from build123d import *

# Parameters (mm, degrees)
F1_DEPTH = 1.5
F3_DEPTH = 25
F4_R     = 0.5
F5_DEPTH = 2.5


# Not quite as in the source:
# - a feature names something its author has since deleted; it is built from what else it names


with BuildPart() as f1:
    # F0 (on Top) → F1 (new body)
    with BuildSketch(Plane.XY):
        Polygon((-37.5444034434, -27.2088618949), (12.4555965566, -35.5019792914), (22.4555965566, -35.5019792914), (22.4555965566, -18.9157444984), (12.4555965566, -18.9157444984), align=None)
    extrude(amount=F1_DEPTH)

    # F2 (on face) → F3 (join)
    with BuildSketch(Plane.XY.offset(1.5)):
        Polygon((-37.5444034434, -27.2088618949), (-1.9112733802, -33.1190565113), (-1.9112733802, -31.1190565113), (-25.486211666, -27.2088618949), (-1.9112733802, -23.2986672785), (-1.9112733802, -21.2986672785), align=None)
    extrude(amount=F3_DEPTH)

    # F4 (on face) → F5 (join)
    with BuildSketch(Plane.XY.offset(1.5)):
        with Locations((17.4555965566, -27.2088618949)):
            Circle(F4_R)
    extrude(amount=F5_DEPTH)


solid = f1.part
Model file for the job. Use its own axes, mm. A direction names the side the tool comes from. Give positions to 0.01 mm unless a question says otherwise; leave off trailing zeros. Write each loop counter-clockwise with the first axis right and the second up, starting at its lowest first coordinate (ties: lowest second). Pieces come first, ordered by that corner, then holes. Notation, with made-up numbers: (-13, 12) -> (11, 12) arc R17 ccw to (11, 27) -> close; hole circle Ø4 at (39, 70). An arc over 180 degrees is marked (long way). Write item = value, one per line.
(1) Slice it at A-A, the plane z = 10.25. Give the cut face in (x, y), then the cut area to 3 significant figures.
Determined:
outline = (-37.54, -27.21) -> (-1.91, -33.12) -> (-1.91, -31.12) -> (-25.49, -27.21) -> (-1.91, -23.3) -> (-1.91, -21.3) -> close
area = 118 mm2
(2) Probe line 1 along Z through (x, y) = (16.5, -34.5); line 2 along Y through (x, z) = (-15, 10.25); line 3 along Y through (x, z) = (-7.5, 10.5). List the from-to ranges inside material, lowest first.
Determined:
line_1 = 0 to 1.5
line_2 = -30.95 to -28.95, -25.47 to -23.47
line_3 = -32.19 to -30.19, -24.23 to -22.23
(3) Mould opens along Y. For faces 1 (the face through (22.456, -27, 1)), 2 (the face through (-13.53, -29.19, 13.82)), 3 (the face through (-18.45, -30.376, 13.064)), 4 (the face through (18, -18.916, 1)) say: released by +Y, released by -Y, zero draft, split by the parting line, or undercut.
Determined:
face_1 = zero draft
face_2 = undercut
face_3 = released by -Y
face_4 = released by +Y
(4) Slice it at D-D, the plane x = -5. Give the cut face in (y, z), then the cut area to 3 significant figures.
Determined:
outline = (-32.61, 0) -> (-21.81, 0) -> (-21.81, 26.5) -> (-23.81, 26.5) -> (-23.81, 1.5) -> (-30.61, 1.5) -> (-30.61, 26.5) -> (-32.61, 26.5) -> close
area = 116 mm2
(5) Slice it at B-B, the plane x = -18. Give the cut face in (y, z), then the cut area to 3 significant figures.
Determined:
outline = (-30.45, 0) -> (-23.97, 0) -> (-23.97, 26.5) -> (-25.97, 26.5) -> (-25.97, 1.5) -> (-28.45, 1.5) -> (-28.45, 26.5) -> (-30.45, 26.5) -> close
area = 110 mm2
(6) Tool access for faces 5 (the face through (-1.911, -32, 14)), 6 (the face through (3, -27, 1.5)), 7 (the face through (17, -35.502, 1)): list every direction of +Z, -Z, +X, -X, +Y, -Y with a clear straight run to the whole face (end or side of a thin tool).
Determined:
face_5 = +Z, +X, +Y, -Y
face_6 = +Z
face_7 = +Z, -Z, +X, -X, -Y
(7) Slice it at C-C, the plane y = -24.25. Give the cut face in (x, z).
Determined:
outline = (-19.71, 0) -> (22.46, 0) -> (22.46, 1.5) -> (-7.65, 1.5) -> (-7.65, 26.5) -> (-19.71, 26.5) -> close
(8) Flat gauge pins, fed straight in: P1, Ø12, axis at x = -28.5, z = 3.5, coming from the -Y side; P2, Ø1, axis at y = -32, z = 15.5, coming from the +X side; P3, Ø8, axis at x = -4, z = 6, coming from the +Y side. Where does each tip first touch, or does it go through?
Determined:
P1 = -29.7
P2 = -1.91
P3 = -21.3
